```python
from build123d import *

# Parameters (mm, degrees)
F0_W     = 34
F0_H     = 3.5
F1_DEPTH = 5
F2_R     = 0.5
F3_DEPTH = 48


with BuildPart() as f1:
    # F0 (on Top) → F1 (new body)
    with BuildSketch(Plane.XY):
        with BuildLine():
            ThreePointArc((0, 2), (0.585786, 0.585786), (2, 0))
            Line((2, 0), (38, 0))
            ThreePointArc((38, 0), (39.414214, 0.585786), (40, 2))
            Line((40, 2), (40, 108))
            ThreePointArc((40, 108), (39.414214, 109.414214), (38, 110))
            Line((38, 110), (2, 110))
            ThreePointArc((2, 110), (0.585786, 109.414214), (0, 108))
            Line((0, 108), (0, 2))
        make_face()
        Polygon((37, 2.5), (3, 2.5), (3, 6), (3, 16), (3, 19.5), (37, 19.5), (37, 16), (37, 6), align=None, mode=Mode.SUBTRACT)
        Polygon((3, 38), (3, 41.5), (37, 41.5), (37, 38), (37, 28), (37, 24.5), (3, 24.5), (3, 28), align=None, mode=Mode.SUBTRACT)
        Polygon((3, 60), (3, 63.5), (37, 63.5), (37, 60), (37, 50), (37, 46.5), (3, 46.5), (3, 50), align=None, mode=Mode.SUBTRACT)
        Polygon((3, 82), (3, 85.5), (37, 85.5), (37, 82), (37, 72), (37, 68.5), (3, 68.5), (3, 72), align=None, mode=Mode.SUBTRACT)
        Polygon((3, 104), (3, 107.5), (37, 107.5), (37, 104), (37, 94), (37, 90.5), (3, 90.5), (3, 94), align=None, mode=Mode.SUBTRACT)
        with Locations((20, 17.75)):
            Rectangle(F0_W, F0_H)
        with Locations((20, 39.75)):
            Rectangle(F0_W, F0_H)
        with Locations((20, 61.75)):
            Rectangle(F0_W, F0_H)
        with Locations((20, 83.75)):
            Rectangle(F0_W, F0_H)
        with Locations((20, 105.75)):
            Rectangle(F0_W, F0_H)
        with Locations((20, 92.25)):
            Rectangle(F0_W, F0_H)
        with Locations((20, 70.25)):
            Rectangle(F0_W, F0_H)
        with Locations((20, 48.25)):
            Rectangle(F0_W, F0_H)
        with Locations((20, 26.25)):
            Rectangle(F0_W, F0_H)
        with Locations((20, 4.25)):
            Rectangle(F0_W, F0_H)
    extrude(amount=F1_DEPTH)

    # F2
    f2_edges = [f1.edges().sort_by_distance(p)[0] for p in [
        (3, 28, 2.5),
        (3, 6, 2.5),
        (3, 50, 2.5),
        (3, 72, 2.5),
        (3, 94, 2.5),
        (3, 104, 2.5),
        (3, 82, 2.5),
        (3, 60, 2.5),
        (3, 38, 2.5),
        (3, 16, 2.5),
        (37, 104, 2.5),
        (37, 82, 2.5),
        (37, 60, 2.5),
        (37, 38, 2.5),
        (37, 16, 2.5),
        (37, 6, 2.5),
        (37, 28, 2.5),
        (37, 50, 2.5),
        (37, 72, 2.5),
        (37, 94, 2.5),
    ]]
    fillet(f2_edges, radius=F2_R)

    # F0 (on Top) → F3 (join)
    with BuildSketch(Plane.XY):
        with BuildLine():
            ThreePointArc((0, 2), (0.585786, 0.585786), (2, 0))
            Line((2, 0), (38, 0))
            ThreePointArc((38, 0), (39.414214, 0.585786), (40, 2))
            Line((40, 2), (40, 108))
            ThreePointArc((40, 108), (39.414214, 109.414214), (38, 110))
            Line((38, 110), (2, 110))
            ThreePointArc((2, 110), (0.585786, 109.414214), (0, 108))
            Line((0, 108), (0, 2))
        make_face()
        Polygon((37, 2.5), (3, 2.5), (3, 6), (3, 16), (3, 19.5), (37, 19.5), (37, 16), (37, 6), align=None, mode=Mode.SUBTRACT)
        Polygon((3, 38), (3, 41.5), (37, 41.5), (37, 38), (37, 28), (37, 24.5), (3, 24.5), (3, 28), align=None, mode=Mode.SUBTRACT)
        Polygon((3, 60), (3, 63.5), (37, 63.5), (37, 60), (37, 50), (37, 46.5), (3, 46.5), (3, 50), align=None, mode=Mode.SUBTRACT)
        Polygon((3, 82), (3, 85.5), (37, 85.5), (37, 82), (37, 72), (37, 68.5), (3, 68.5), (3, 72), align=None, mode=Mode.SUBTRACT)
        Polygon((3, 104), (3, 107.5), (37, 107.5), (37, 104), (37, 94), (37, 90.5), (3, 90.5), (3, 94), align=None, mode=Mode.SUBTRACT)
    extrude(amount=F3_DEPTH)


solid = f1.part
```
Verification items for the finished model (mm, model axes). A direction names the side the tool comes from. Round coordinates to 2 decimals unless told otherwise and drop trailing zeros. Write each loop counter-clockwise with the first axis right and the second up, starting at its lowest first coordinate (ties: lowest second). Pieces come first, ordered by that corner, then holes. Notation, with made-up numbers: (21.25, 11.25) -> (56.25, 11.25) arc R28 cw to (56.25, 32.25) -> close; hole circle Ø5 at (7, 1.25). An arc over 180 degrees is marked (long way). Write each question's results on one line, items separated by ' | '.
Q1. Sectioned sample at B-B, the plane y = 79. Record the boundary of the cut face in (x, z), and give its area (3 significant figures).
Derived:
outline: (0, 0) -> (3, 0) -> (3, 48) -> (0, 48) -> close; (37, 0) -> (40, 0) -> (40, 48) -> (37, 48) -> close | area: 288 mm²
Q2. Access from +Z, -Z, +X, -X, +Y, -Y to the whole of each face (thin tool, end or side, straight path). Record for faces 5 (the face through (20, 18, 5)), 6 (the face through (20, 68, 0)), 7 (the face through (20, 16, 2)).
Derived:
face 5: +Z | face 6: -Z, +X, -X, +Y, -Y | face 7: +Z, -Z
Q3. Draft check along X on faces 1 (the face through (40, 54, 24)), 2 (the face through (20, 110, 24)), 3 (the face through (37, 11, 24)), 4 (the face through (20, 46.5, 26)). Enter one of: released by +X, released by -X, zero draft, split by the parting line, or undercut.
Derived:
face 1: released by +X | face 2: zero draft | face 3: undercut | face 4: undercut
Q4. Sectioned sample at A-A, the plane z = 17. Record the boundary of the cut face in (x, y).
Derived:
outline: (0, 2) arc R2 ccw to (2, 0) -> (38, 0) arc R2 ccw to (40, 2) -> (40, 108) arc R2 ccw to (38, 110) -> (2, 110) arc R2 ccw to (0, 108) -> close; hole (3, 2.5) -> (37, 2.5) -> (37, 19.5) -> (3, 19.5) -> close; hole (3, 24.5) -> (37, 24.5) -> (37, 41.5) -> (3, 41.5) -> close; hole (3, 46.5) -> (37, 46.5) -> (37, 63.5) -> (3, 63.5) -> close; hole (3, 68.5) -> (37, 68.5) -> (37, 85.5) -> (3, 85.5) -> close; hole (3, 90.5) -> (37, 90.5) -> (37, 107.5) -> (3, 107.5) -> close
Q5. Thickness scan on probe 1 along Y at (x, z) = (24.5, 43.5); probe 2 along Y at (x, z) = (10.5, 3.5); probe 3 along X at (y, z) = (91.5, 40.5). Record the ranges inside material, lowest first.
Derived:
probe 1: y = 0 to 2.5, 19.5 to 24.5, 41.5 to 46.5, 63.5 to 68.5, 85.5 to 90.5, 107.5 to 110 | probe 2: y = 0 to 6, 16 to 28, 38 to 50, 60 to 72, 82 to 94, 104 to 110 | probe 3: x = 0 to 3, 37 to 40
Q6. Sectioned sample at C-C, the plane x = 29. Give the number of separate pieces and of enclosed holes in the cut face, and give its area (4 significant figures).
Derived:
separate pieces: 6 | enclosed holes: 0 | area: 1,375 mm²
Q7. Go/stop test with a flat-tipped pin: pin 1 Ø4.5 at (x, y) = (24, 83) entering from +Z. Record where the tip stops, or that it passes through.
Derived:
pin 1: stops at z = 5
